```python
from build123d import *

# Parameters (mm, degrees)
BOSS_EXTRUDE1_DEPTH = 19.05


with BuildPart() as part:
    # Sketch1 → Boss-Extrude1 (new body)
    with BuildSketch(Plane(origin=(0, 0, 0), x_dir=(1, 0, 0), z_dir=(0, 1, 0))):
        with BuildLine():
            Line((-19.05, 142.604993733), (-19.05, 163.473390846))
            ThreePointArc((-19.05, 163.473390846), (14.378745185, 237.368638748), (91.949229987, 261.050035552))
            ThreePointArc((91.949229987, 261.050035552), (112.649599057, 236.081870166), (89.206052596, 213.669492074))
            ThreePointArc((89.206052596, 213.669492074), (39.543801874, 192.535031386), (19.05, 142.604993733))
            Line((19.05, 142.604993733), (19.05, 0))
            Line((19.05, 0), (-19.05, 0))
            Line((-19.05, 0), (-19.05, 142.604993733))
        make_face()
    extrude(amount=BOSS_EXTRUDE1_DEPTH)


solid = part.part
```
CAD build for the part. Positions are in the model's coordinates, mm. A direction names the side the tool comes from. Round coordinates to 2 decimals unless told otherwise and drop trailing zeros. Write each loop counter-clockwise with the first axis right and the second up, starting at its lowest first coordinate (ties: lowest second). Pieces come first, ordered by that corner, then holes. Notation, with made-up numbers: (-4, 19) - (36, 19) arc R12 cw to (36, 34) - close; hole circle Ø9 at (-15.75, 32). An arc over 180 degrees is marked (long way). Return JSON: item names as keys, results as strings. Group by question number.
Item 1: Band-saw the part on B-B on z = -36.5. List the corners of the cut face in (x, y).
Item 2: Flat gauge pins, fed straight in: pin 1 Ø10 at (x, y) = (88, 13) entering from +Z; pin 2 Ø3 at (y, z) = (17, -182) entering from -X; pin 3 Ø1 at (y, z) = (8.5, -210.5) entering from -X. Where does each tip first touch, or does it go through?
Item 3: Band-saw the part on C-C on x = 38. List the corners of the cut face in (y, z), plus the area to 3 significant figures.
Item 4: Probe probe 1 along X at (y, z) = (7, -62); probe 2 along Z at (x, y) = (3, 6.25). List the from-to ranges inside material, lowest first.
Item 5: 3-axis set-ups, long thin cutter, end or side, ignore diameter. For faces 1 (the face through (19.05, 9, -72)), 2 (the face through (0, 9, 0)): which of +Z, -Z, +X, -X, +Y, -Y reach the whole face in a straight line?
Resolved:
{
 "1": {"outline": "(-19.05, 0) - (19.05, 0) - (19.05, 19.05) - (-19.05, 19.05) - close"},
 "2": {"pin 1": "stops at z = -213.32", "pin 2": "stops at x = -17.57", "pin 3": "stops at x = -7.35"},
 "3": {"outline": "(0, -252.76) - (19.05, -252.76) - (19.05, -190.92) - (0, -190.92) - close", "area": "1,180 mm²"},
 "4": {"probe 1": "x = -19.05 to 19.05", "probe 2": "z = -225.54 to 0"},
 "5": {"face 1": "+Z, +X, +Y, -Y", "face 2": "+Z, +X, -X, +Y, -Y"}
}
